```python
from build123d import *

# Parameters (mm, degrees)
EXTRUDE_1_DEPTH = 10


with BuildPart() as part:
    # Sketch 1 → Extrude 1 (new body)
    with BuildSketch(Plane.XY):
        with BuildLine():
            Line((2.620879352, -3.464979969), (0, 0))
            Line((0, 0), (-0.775570302, 0))
            Line((-0.775570302, 0), (4.99793245, -10.000000104))
            ThreePointArc((4.99793245, -10.000000104), (3.523202171, -6.836593995), (2.620879352, -3.464979969))
        make_face()
        with BuildLine():
            Line((12.110887706, -16.011413604), (8.122108144, -10.737976934))
            Line((8.122108144, -10.737976934), (2.620879352, -3.464979969))
            ThreePointArc((2.620879352, -3.464979969), (3.523202171, -6.836593995), (4.99793245, -10.000000104))
            ThreePointArc((4.99793245, -10.000000104), (8.091530745, -14.056850281), (12.110887706, -17.199007723))
            Line((12.110887706, -17.199007723), (12.110887706, -16.011413604))
        make_face()
        with BuildLine():
            ThreePointArc((8.122108144, -10.737976934), (5.443389127, -5.663271346), (4.518440465, 0))
            Line((4.518440465, 0), (2.318440465, 0))
            ThreePointArc((2.318440465, 0), (2.394193651, -1.739077016), (2.620879352, -3.464979969))
            Line((2.620879352, -3.464979969), (8.122108144, -10.737976934))
        make_face()
        with BuildLine():
            Line((12.110887706, -16.011413604), (12.110887706, -14.582382064))
            ThreePointArc((12.110887706, -14.582382064), (9.966021089, -12.816307407), (8.122108144, -10.737976934))
            Line((8.122108144, -10.737976934), (12.110887706, -16.011413604))
        make_face()
        with BuildLine():
            Line((2.318440465, 0), (0, 0))
            Line((0, 0), (2.620879352, -3.464979969))
            ThreePointArc((2.620879352, -3.464979969), (2.394193651, -1.739077016), (2.318440465, 0))
        make_face()
        with BuildLine():
            ThreePointArc((2.318440465, 0), (2.394193651, 1.739077016), (2.620879352, 3.464979969))
            Line((2.620879352, 3.464979969), (0, 0))
            Line((0, 0), (2.318440465, 0))
        make_face()
        with BuildLine():
            Line((0, 0), (2.620879352, 3.464979969))
            ThreePointArc((2.620879352, 3.464979969), (3.523202169, 6.83659399), (4.997932444, 10.000000095))
            Line((4.997932444, 10.000000095), (-0.775570302, 0))
            Line((-0.775570302, 0), (0, 0))
        make_face()
        with BuildLine():
            ThreePointArc((4.518440465, 0), (5.44338905, 5.663271114), (8.122107849, 10.737976543))
            Line((8.122107849, 10.737976543), (2.620879352, 3.464979969))
            ThreePointArc((2.620879352, 3.464979969), (2.394193651, 1.739077016), (2.318440465, 0))
            Line((2.318440465, 0), (4.518440465, 0))
        make_face()
        with BuildLine():
            Line((8.122107849, 10.737976543), (12.110887706, 16.011413604))
            Line((12.110887706, 16.011413604), (12.110887706, 17.199007723))
            ThreePointArc((12.110887706, 17.199007723), (8.091530741, 14.056850277), (4.997932444, 10.000000095))
            ThreePointArc((4.997932444, 10.000000095), (3.523202169, 6.83659399), (2.620879352, 3.464979969))
            Line((2.620879352, 3.464979969), (8.122107849, 10.737976543))
        make_face()
        with BuildLine():
            Line((12.110887706, 14.582382064), (12.110887706, 16.011413604))
            Line((12.110887706, 16.011413604), (8.122107849, 10.737976543))
            ThreePointArc((8.122107849, 10.737976543), (9.966020913, 12.816307237), (12.110887706, 14.582382064))
        make_face()
    extrude(amount=EXTRUDE_1_DEPTH)

    # Sketch 2 → Cut-Revolve 1 (revolve, cut)
    with BuildSketch(Plane(origin=(0, 0, 0), x_dir=(0, 0, -1), z_dir=(0, -1, 0))):
        Polygon((0, 22.318440465), (0, 4.518440465), (-10, 3.831448348), (-10, 22.318440465), align=None)
    revolve(axis=Axis((22.318440465, 0, 18.306126046), (0, 0, -1)), mode=Mode.SUBTRACT)


solid = part.part
```
Geometry: final body of the model. Coordinates: model frame, mm. Round coordinates to 2 decimals unless told otherwise and drop trailing zeros. Order: outer loops, then holes, each group sorted by start corner. A loop starts at its lowest first (then second) coordinate and runs counter-clockwise, first axis right, second up. Notation, with made-up numbers: (59.5, -1.75) -> (68.5, -1.75) arc R30 cw to (68.5, 27.25) -> close; hole circle Ø7 at (8.25, -10). An arc over 180 degrees is marked (long way). Write each question's results on one line, items separated by ' | '.
Q1. Section query A-A (z = 8). Output: boundary loops of the cut face in (x, y).
Response values:
outline: (-0.78, 0) -> (5, -10) arc R20 ccw to (12.11, -17.2) -> (12.11, -15.25) arc R18.35 cw to (12.11, 15.25) -> (12.11, 17.2) arc R20 ccw to (5, 10) -> close
Q2. Section query C-C (z = 5). Output: boundary loops of the cut face in (x, y), and give its area (3 significant figures).
Response values:
outline: (-0.78, 0) -> (5, -10) arc R20 ccw to (12.11, -17.2) -> (12.11, -15) arc R18.14 cw to (12.11, 15) -> (12.11, 17.2) arc R20 ccw to (5, 10) -> close | area: 92.7 mm²
Q3. Pin query (flat end, axial travel): pin 1 Ø2 at (x, z) = (9, 7.5) entering from -Y; pin 2 Ø1 at (x, z) = (4.5, 5.5) entering from -Y. Return the tip coordinate at first contact, or that it passes through.
Response values:
pin 1: y = -15.76 | pin 2: y = -10
Q4. Section query D-D (x = 3.5). Output: boundary loops of the cut face in (y, z), and give its area (3 significant figures).
Response values:
outline: (-7.41, 0) -> (7.41, 0) -> (7.41, 10) -> (-7.41, 10) -> close | area: 148 mm²
Q5. Ray query, line 1 along Y through (x, z) = (10.5, 6); line 2 along Y through (x, z) = (10.5, 7); line 3 along X through (y, z) = (10.5, 6.75). Return the intervals inside material, ascending.
Response values:
line 1: -16.13 to -13.86, 13.86 to 16.13 | line 2: -16.13 to -13.95, 13.95 to 16.13 | line 3: 5.3 to 7.37
Q6. Section query B-B (x = 1.25). Output: boundary loops of the cut face in (y, z), and give its area (3 significant figures).
Response values:
outline: (-3.51, 0) -> (3.51, 0) -> (3.51, 10) -> (-3.51, 10) -> close | area: 70.2 mm²
